Geometry check sheet. Reference: drawing and pictorial views, mm from the part's lowest x, y, z. A direction names the side the tool comes from. Coordinates: 2 decimals unless noted, no trailing zeros. Loops run counter-clockwise (first coordinate to the right, second up) from the corner with the lowest first, then second, coordinate; pieces in that order, holes last. Notation, with made-up numbers: (-31, 10) -> (6, 10) arc R24 cw to (6, 49) -> close; hole circle Ø3 at (-2.5, -1.5). An arc over 180 degrees is marked (long way). Use one line per item in the form item = value.
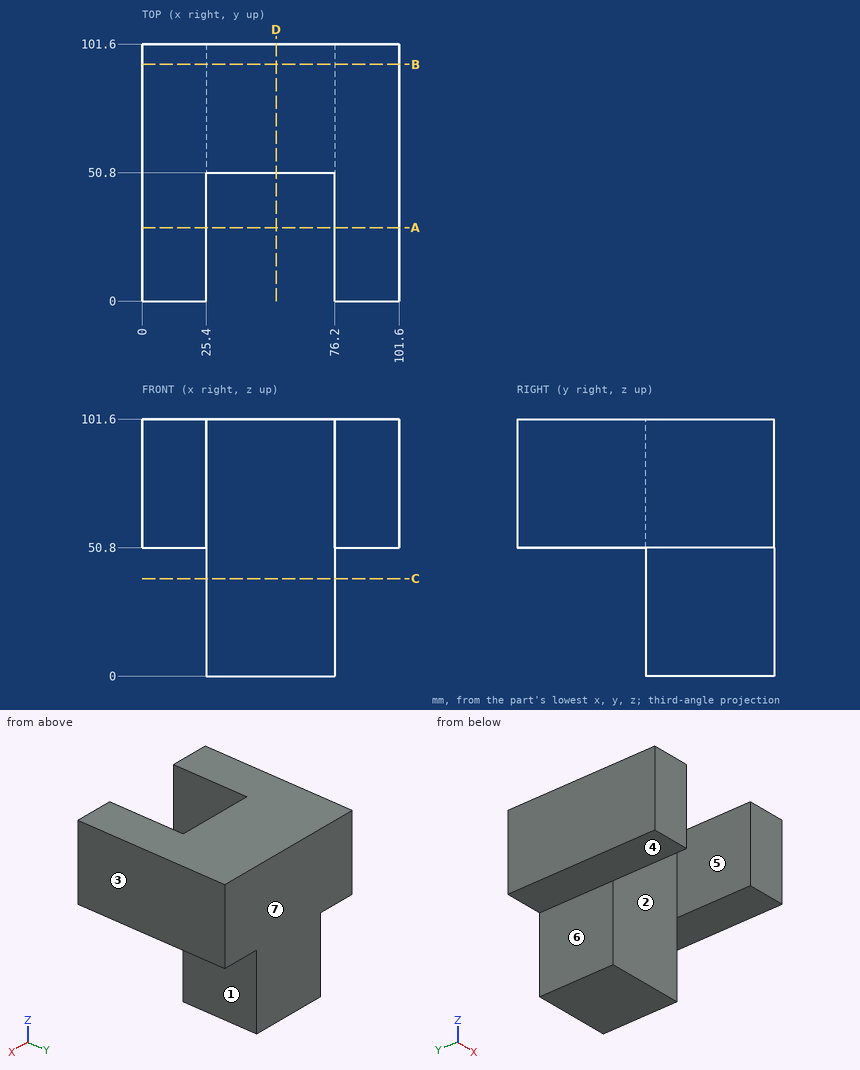
(1) Section check A-A, the plane y = 29. Record the boundary of the cut face in (x, z).
Established:
outline = (0, 50.8) -> (25.4, 50.8) -> (25.4, 101.6) -> (0, 101.6) -> close; (76.2, 50.8) -> (101.6, 50.8) -> (101.6, 101.6) -> (76.2, 101.6) -> close
(2) Scan lines: line 1 along X through (y, z) = (45, 66.5); line 2 along X through (y, z) = (64, 22.5); line 3 along Y through (x, z) = (41, 65). Record each from-to range of solid material in increasing order.
Established:
line_1 = 0 to 25.4, 76.2 to 101.6
line_2 = 25.4 to 76.2
line_3 = 50.8 to 101.6
(3) Go/stop test with flat-tipped pins: P1, Ø7.5, axis at x = 17.5, y = 42.5, coming from the -Z side; P2, Ø15, axis at x = 49, z = 63.5, coming from the -Y side; P3, Ø2, axis at y = 77.5, z = 48, coming from the -X side. Record where each tip stops, or that it passes through.
Established:
P1 = 50.8
P2 = 50.8
P3 = 25.4
(4) Section check D-D, the plane x = 53. Record the boundary of the cut face in (y, z), plus the area to 3 significant figures.
Established:
outline = (50.8, 0) -> (101.6, 0) -> (101.6, 101.6) -> (50.8, 101.6) -> close
area = 5,160 mm²
(5) Section check C-C, the plane z = 38.5. Record the boundary of the cut face in (x, y).
Established:
outline = (25.4, 50.8) -> (76.2, 50.8) -> (76.2, 101.6) -> (25.4, 101.6) -> close
(6) Section check B-B, the plane y = 93.5. Record the boundary of the cut face in (x, z), plus the area to 3 significant figures.
Established:
outline = (0, 50.8) -> (25.4, 50.8) -> (25.4, 0) -> (76.2, 0) -> (76.2, 50.8) -> (101.6, 50.8) -> (101.6, 101.6) -> (0, 101.6) -> close
area = 7,740 mm²
(7) Mould release check, pull along X, two halves, no side actions. Record for the marked faces 5, 6 and 7: +X half, -X half, draft (parallel to the pull), parting line (faces both ways), or undercut.
Established:
face_5 = undercut
face_6 = -X half
face_7 = draft
(8) Tool access check on the marked faces 1, 2, 3 and 4. Record the directions out of +Z, -Z, +X, -X, +Y, -Y that give a thin tool (end or side, any length) a straight path to the whole face; none if there is none.
Established:
face_1 = -Z, +X, +Y, -Y
face_2 = +Z, -Z, -Y
face_3 = +Z, -Z, +X, +Y, -Y
face_4 = -Z, -X, +Y, -Y
